For this review, take the finished solid that the model builds, in its own axes (mm). A direction names the side the tool comes from. Coordinates: 2 decimals unless noted, no trailing zeros. Write each loop counter-clockwise with the first axis right and the second up, starting at its lowest first coordinate (ties: lowest second). Pieces come first, ordered by that corner, then holes. Notation, with made-up numbers: (-27, 6) - (-22, 6) arc R22 cw to (-22, 35) - close; hole circle Ø7 at (67, -25.75). An arc over 180 degrees is marked (long way). Write each question's results on one line, items separated by ' | '.
from build123d import *

# Parameters (mm, degrees)
ESBO_O1_W                  = 100
ESBO_O1_H                  = 43
RESSALTO_EXTRUS_O1_DEPTH   = 1.5
ESBO_O2_R                  = 1.5
CORTE_EXTRUS_O1_DEPTH      = 55.50917354
CUT_EXTRUDE6_DEPTH         = 55.447222151
CUT_EXTRUDE6_DEPTH_BACK    = 55.447222151
SKETCH7_W                  = 13.5
SKETCH7_H                  = 9.5
SKETCH8_W                  = 3
SKETCH8_H                  = 34.5
BOSS_EXTRUDE1_DEPTH        = 1.5
FILLET3_R                  = 2
FILLET4_R                  = 5
CORTE_GY_VL53L0_DEPTH      = 58.214508649
CORTE_GY_VL53L0_DEPTH_BACK = 58.214508649
CUT_EXTRUDE7_DEPTH         = 58.273466806
CUT_EXTRUDE7_DEPTH_BACK    = 58.273466806


with BuildPart() as part:
    # Esboço1 → Ressalto-extrusão1 (new, symmetric)
    with BuildSketch(Plane.XY):
        Rectangle(ESBO_O1_W, ESBO_O1_H)
    extrude(amount=RESSALTO_EXTRUS_O1_DEPTH, both=True)

    # Esboço2 → Corte-extrusão1 (cut, through all)
    with BuildSketch(Plane.XY.offset(1.5)):
        with Locations((-33, -17)):
            Circle(ESBO_O2_R)
        with Locations(Location((33, -17, 0), (0, 0, 180))):
            Circle(ESBO_O2_R)
        Polygon((-20, -15.5), (-7.5, -15.5), (-7.5, -12.5), (7.5, -12.5), (7.5, -15.5), (20, -15.5), (20, -18.5), (7.5, -18.5), (7.5, -21.5), (-7.5, -21.5), (-7.5, -18.5), (-20, -18.5), align=None)
    extrude(amount=-CORTE_EXTRUS_O1_DEPTH, mode=Mode.SUBTRACT)

    # Sketch7 → Cut-Extrude6 (cut, two sides: drawn at the far end of the back side and taken through both)
    with BuildSketch(Plane.XY.offset(-CUT_EXTRUDE6_DEPTH_BACK)):
        with Locations((22.1, -2.25)):
            Rectangle(SKETCH7_W, SKETCH7_H)
        with Locations((22.1, 11.25)):
            Rectangle(SKETCH7_W, SKETCH7_H)
    extrude(amount=CUT_EXTRUDE6_DEPTH + CUT_EXTRUDE6_DEPTH_BACK, mode=Mode.SUBTRACT)

    # Sketch8 → Boss-Extrude1 (add, symmetric)
    with BuildSketch(Plane.XY):
        with Locations((-51.5, 4.25)):
            Rectangle(SKETCH8_W, SKETCH8_H)
        with Locations((51.5, 4.25)):
            Rectangle(SKETCH8_W, SKETCH8_H)
    extrude(amount=BOSS_EXTRUDE1_DEPTH, both=True)

    # Fillet3
    fillet3_edges = [part.edges().sort_by_distance(p)[0] for p in [
        (-7.5, -21.5, 0),
        (-7.5, -12.5, 0),
        (7.5, -12.5, 0),
        (7.5, -21.5, 0),
    ]]
    fillet(fillet3_edges, radius=FILLET3_R)

    # Fillet4
    fillet4_edges = [part.edges().sort_by_distance(p)[0] for p in [
        (53, 21.5, 0),
        (-53, 21.5, 0),
    ]]
    fillet(fillet4_edges, radius=FILLET4_R)

    # Sketch6 → Corte Gy-VL53L0 (cut, two sides: drawn at the far end of the back side and taken through both)
    with BuildSketch(Plane.XY.offset(-CORTE_GY_VL53L0_DEPTH_BACK)):
        with BuildLine():
            Line((-40.5, 14.030680232), (-40.504337567, 14.030680232))
            ThreePointArc((-40.504337567, 14.030680232), (-40.937350269, 14.280680232), (-40.937350269, 14.780680232))
            Line((-40.937350269, 14.780680232), (-40.36, 15.780680232))
            Line((-40.36, 15.780680232), (-41.93, 18.5))
            Line((-41.93, 18.5), (-45.07, 18.5))
            Line((-45.07, 18.5), (-46.64, 15.780680232))
            Line((-46.64, 15.780680232), (-46.062649731, 14.780680232))
            ThreePointArc((-46.062649731, 14.780680232), (-46.062649731, 14.280680232), (-46.495662433, 14.030680232))
            Line((-46.495662433, 14.030680232), (-48, 14.030680232))
            ThreePointArc((-48, 14.030680232), (-49.414213562, 13.444893794), (-50, 12.030680232))
            Line((-50, 12.030680232), (-50, 0.030680232))
            ThreePointArc((-50, 0.030680232), (-49.414213562, -1.38353333), (-48, -1.969319768))
            Line((-48, -1.969319768), (-46.495662433, -1.969319768))
            ThreePointArc((-46.495662433, -1.969319768), (-46.062649731, -2.219319768), (-46.062649731, -2.719319768))
            Line((-46.062649731, -2.719319768), (-46.64, -3.719319768))
            Line((-46.64, -3.719319768), (-45.07, -6.438639536))
            Line((-45.07, -6.438639536), (-41.93, -6.438639536))
            Line((-41.93, -6.438639536), (-40.36, -3.719319768))
            Line((-40.36, -3.719319768), (-40.937350269, -2.719319768))
            ThreePointArc((-40.937350269, -2.719319768), (-40.937350269, -2.219319768), (-40.504337567, -1.969319768))
            Line((-40.504337567, -1.969319768), (-39, -1.969319768))
            ThreePointArc((-39, -1.969319768), (-37.585786438, -1.38353333), (-37, 0.030680232))
            Line((-37, 0.030680232), (-37, 6.030680232))
            Line((-37, 6.030680232), (-37, 12.030680232))
            ThreePointArc((-37, 12.030680232), (-37.585786438, 13.444893794), (-39, 14.030680232))
            Line((-39, 14.030680232), (-40.5, 14.030680232))
        make_face()
        with BuildLine():
            Line((40.5, 14.030680232), (40.504337567, 14.030680232))
            ThreePointArc((40.504337567, 14.030680232), (40.937350269, 14.280680232), (40.937350269, 14.780680232))
            Line((40.937350269, 14.780680232), (40.36, 15.780680232))
            Line((40.36, 15.780680232), (41.93, 18.5))
            Line((41.93, 18.5), (45.07, 18.5))
            Line((45.07, 18.5), (46.64, 15.780680232))
            Line((46.64, 15.780680232), (46.062649731, 14.780680232))
            ThreePointArc((46.062649731, 14.780680232), (46.062649731, 14.280680232), (46.495662433, 14.030680232))
            Line((46.495662433, 14.030680232), (48, 14.030680232))
            ThreePointArc((48, 14.030680232), (49.414213562, 13.444893794), (50, 12.030680232))
            Line((50, 12.030680232), (50, 0.030680232))
            ThreePointArc((50, 0.030680232), (49.414213562, -1.38353333), (48, -1.969319768))
            Line((48, -1.969319768), (46.495662433, -1.969319768))
            ThreePointArc((46.495662433, -1.969319768), (46.062649731, -2.219319768), (46.062649731, -2.719319768))
            Line((46.062649731, -2.719319768), (46.64, -3.719319768))
            Line((46.64, -3.719319768), (45.07, -6.438639536))
            Line((45.07, -6.438639536), (41.93, -6.438639536))
            Line((41.93, -6.438639536), (40.36, -3.719319768))
            Line((40.36, -3.719319768), (40.937350269, -2.719319768))
            ThreePointArc((40.937350269, -2.719319768), (40.937350269, -2.219319768), (40.504337567, -1.969319768))
            Line((40.504337567, -1.969319768), (39, -1.969319768))
            ThreePointArc((39, -1.969319768), (37.585786438, -1.38353333), (37, 0.030680232))
            Line((37, 0.030680232), (37, 6.030680232))
            Line((37, 6.030680232), (37, 12.030680232))
            ThreePointArc((37, 12.030680232), (37.585786438, 13.444893794), (39, 14.030680232))
            Line((39, 14.030680232), (40.5, 14.030680232))
        make_face()
    extrude(amount=CORTE_GY_VL53L0_DEPTH + CORTE_GY_VL53L0_DEPTH_BACK, mode=Mode.SUBTRACT)

    # Sketch11 → Cut-Extrude7 (cut, two sides: drawn at the far end of the back side and taken through both)
    with BuildSketch(Plane.XY.offset(1.5).offset(-CUT_EXTRUDE7_DEPTH_BACK)):
        with BuildLine():
            Line((-32, 10.2), (-12.78, 10.2))
            ThreePointArc((-12.78, 10.2), (-11.365786438, 9.614213562), (-10.78, 8.2))
            Line((-10.78, 8.2), (-10.78, 3.9))
            ThreePointArc((-10.78, 3.9), (-11.365786438, 2.485786438), (-12.78, 1.9))
            Line((-12.78, 1.9), (-32, 1.9))
            ThreePointArc((-32, 1.9), (-33.414213562, 2.485786438), (-34, 3.9))
            Line((-34, 3.9), (-34, 8.2))
            ThreePointArc((-34, 8.2), (-33.414213562, 9.614213562), (-32, 10.2))
        make_face()
    extrude(amount=CUT_EXTRUDE7_DEPTH + CUT_EXTRUDE7_DEPTH_BACK, mode=Mode.SUBTRACT)


solid = part.part
Q1. For faces 5 (the face through (-20, -17, 0)), 6 (the face through (6.93, -13.1, -0.02)), 7 (the face through (-1, 21.5, 0)), list the 3-axis set-ups (+Z, -Z, +X, -X, +Y, -Y) from which the entire face can be reached by the end or side of a thin tool; tool diameter is ignored.
Results found:
face 5: +Z, -Z | face 6: +Z, -Z, -Y | face 7: +Z, -Z, +X, -X, +Y
Q2. Take a section at B-B on x = -14.5. State the section outline as (y, z) points, plus the area to 3 significant figures.
Results found:
outline: (-21.5, -1.5) - (-18.5, -1.5) - (-18.5, 1.5) - (-21.5, 1.5) - close; (-15.5, -1.5) - (1.9, -1.5) - (1.9, 1.5) - (-15.5, 1.5) - close; (10.2, -1.5) - (21.5, -1.5) - (21.5, 1.5) - (10.2, 1.5) - close | area: 95.1 mm2
Q3. Take a section at C-C on x = 33. State the section outline as (y, z) points.
Results found:
outline: (-21.5, -1.5) - (-18.5, -1.5) - (-18.5, 1.5) - (-21.5, 1.5) - close; (-15.5, -1.5) - (21.5, -1.5) - (21.5, 1.5) - (-15.5, 1.5) - close
Q4. For pin 1 (1.1 mm diameter, centred on y = -15, z = -0.5, fed in from +X); pin 2 (5 mm diameter, centred on x = 41.5, y = 13, fed in from -Z); pin 3 (0.8 mm diameter, centred on y = -15, z = 0, fed in from -X), all flat-tipped, find the tip position at first contact; note any pin that passes through.
Results found:
pin 1: x = 50 | pin 2: z = -1.5 | pin 3: x = -50
Q5. Wall thickness on line 1 along Y through (x, z) = (19, -0.25); line 2 along X through (y, z) = (0.5, 0.6); line 3 along Y through (x, z) = (40, -0.8): over which ranges is each line inside the solid? List them lowest first. Write a range as from..to.
Results found:
line 1: -21.5..-18.5, -15.5..-7, 2.5..6.5, 16..21.5 | line 2: -53..-50, -37..15.35, 28.85..37, 50..53 | line 3: -21.5..-1.97, 14.03..21.5
Q6. Take a section at A-A on y = -17. State the section outline as (x, z) points, plus the area to 3 significant figures.
Results found:
outline: (-50, -1.5) - (-34.5, -1.5) - (-34.5, 1.5) - (-50, 1.5) - close; (-31.5, -1.5) - (-20, -1.5) - (-20, 1.5) - (-31.5, 1.5) - close; (20, -1.5) - (31.5, -1.5) - (31.5, 1.5) - (20, 1.5) - close; (34.5, -1.5) - (50, -1.5) - (50, 1.5) - (34.5, 1.5) - close | area: 162 mm2
Q7. Take a section at D-D on z = -0.8. State how many separate pieces and enclosed holes the cut face has, plus the area to 3 significant figures.
Results found:
separate pieces: 1 | enclosed holes: 7 | area: 3,330 mm2
Q8. Mouldability with a two-part tool opening along X and no side actions: class faces 1 (the face through (-30, -21.5, 0)), 2 (the face through (-11.38, 9.63, -0.02)), 3 (the face through (22, 2.5, 0)), 4 (the face through (51.5, 20.07, -0.02)) as pulls with the +X half, pulls with the -X half, needs draft (parallel to the pull), parting line crosses it, or undercut.
Results found:
face 1: needs draft | face 2: undercut | face 3: undercut | face 4: pulls with the +X half
